Build history of the part. All positions in model axes, mm. A direction names the side the tool comes from. Coordinates: 2 decimals unless noted, no trailing zeros. Order: outer loops, then holes, each group sorted by start corner. A loop starts at its lowest first (then second) coordinate and runs counter-clockwise, first axis right, second up. Notation, with made-up numbers: (28.5, 6) - (77.5, 6) arc R14 ccw to (77.5, 25) - close; hole circle Ø11 at (17.25, -23.5). An arc over 180 degrees is marked (long way). One line per item, written item: value.
from build123d import *

# Parameters (mm, degrees)
F0_W     = 25.4
F0_H     = 50.8
F0_W_2   = 20.32
F0_H_2   = 45.72
F1_DEPTH = 304.8
F2_R     = 14.2875
F2_R_2   = 3.3782
F2_R_3   = 2.4892
F3_DEPTH = 25.4
F4_R     = 2.4892
F5_DEPTH = 50.801


with BuildPart() as f1:
    # F0 (on Top) → F1 (new body)
    with BuildSketch(Plane.XY):
        with Locations((12.7, -25.4)):
            Rectangle(F0_W, F0_H)
        with Locations((12.7, -25.4)):
            Rectangle(F0_W_2, F0_H_2, mode=Mode.SUBTRACT)
    extrude(amount=F1_DEPTH)

    # F2 (on face) → F3 (cut)
    with BuildSketch(Plane.YZ.offset(25.4)):
        with Locations((-25.4, 254)):
            Circle(F2_R)
        with Locations((-38.1, 38.1)):
            Circle(F2_R_2)
        with Locations((-38.1, 12.7)):
            Circle(F2_R_2)
        with Locations((-12.7, 38.1)):
            Circle(F2_R_2)
        with Locations((-12.7, 12.7)):
            Circle(F2_R_2)
        with BuildLine():
            ThreePointArc((-4.950288, 167.27389), (-8.392063, 169.573611), (-9.199618, 165.51376))
            ThreePointArc((-9.199618, 165.51376), (-6.486912, 164.974169), (-4.950288, 167.27389))
        make_face()
        with Locations((-43.360512, 131.352866)):
            Circle(F2_R_3)
        with BuildLine():
            Line((-25.4, 149.313378), (-11.1125, 149.313378))
            ThreePointArc((-11.1125, 149.313378), (-12.200071, 154.780968), (-15.297212, 159.416166))
            Line((-15.297212, 159.416166), (-25.4, 149.313378))
        make_face()
        with BuildLine():
            ThreePointArc((-15.297212, 159.416166), (-38.599929, 143.845789), (-11.1125, 149.313378))
            Line((-11.1125, 149.313378), (-25.4, 149.313378))
            Line((-25.4, 149.313378), (-15.297212, 159.416166))
        make_face()
    extrude(amount=-F3_DEPTH, mode=Mode.SUBTRACT)

    # F4 (on face) → F5 (cut, through all)
    with BuildSketch(Plane.XZ.offset(50.8)):
        with Locations((12.7, 292.1)):
            Circle(F4_R)
        with Locations((12.7, 266.7)):
            Circle(F4_R)
        with Locations((12.7, 241.3)):
            Circle(F4_R)
        with Locations((12.7, 215.9)):
            Circle(F4_R)
        with Locations((12.7, 190.5)):
            Circle(F4_R)
        with Locations((12.7, 165.1)):
            Circle(F4_R)
    extrude(amount=-F5_DEPTH, mode=Mode.SUBTRACT)


solid = f1.part
1. 3-axis set-ups, long thin cutter, end or side, ignore diameter. For faces 5 (the face through (13.849, -49.548, 213.692)), 6 (the face through (22.86, -41, 150)): which of +Z, -Z, +X, -X, +Y, -Y reach the whole face in a straight line?
Values found:
face 5: +Y, -Y
face 6: +Z, -Z
2. Probe line 1 along Z through (x, y) = (24.3, -25.4); line 2 along X through (y, z) = (-35, 240); line 3 along Z through (x, y) = (0.75, -12.7). List the from-to ranges inside material, lowest first.
Values found:
line 1: z = 0 to 135.03, 163.6 to 239.71, 268.29 to 304.8
line 2: x = 0 to 2.54, 22.86 to 25.4
line 3: z = 0 to 9.32, 16.08 to 34.72, 41.48 to 142.77, 155.86 to 247.45, 260.55 to 304.8
3. Band-saw the part on C-C, the plane z = 254. Give the cut face in (x, y).
Values found:
outline: (0, -50.8) - (25.4, -50.8) - (25.4, -39.69) - (22.86, -39.69) - (22.86, -48.26) - (2.54, -48.26) - (2.54, -39.69) - (0, -39.69) - close; (0, -11.11) - (2.54, -11.11) - (2.54, -2.54) - (22.86, -2.54) - (22.86, -11.11) - (25.4, -11.11) - (25.4, 0) - (0, 0) - close
4. Band-saw the part on B-B, the plane y = -25.4. Give the cut face in (x, z), and give its area (3 significant figures).
Values found:
outline: (0, 0) - (2.54, 0) - (2.54, 135.03) - (0, 135.03) - close; (0, 163.6) - (2.54, 163.6) - (2.54, 239.71) - (0, 239.71) - close; (0, 268.29) - (2.54, 268.29) - (2.54, 304.8) - (0, 304.8) - close; (22.86, 0) - (25.4, 0) - (25.4, 135.03) - (22.86, 135.03) - close; (22.86, 163.6) - (25.4, 163.6) - (25.4, 239.71) - (22.86, 239.71) - close; (22.86, 268.29) - (25.4, 268.29) - (25.4, 304.8) - (22.86, 304.8) - close
area: 1,260 mm2
5. Two-plate mould, pull along Y, no slides. Class faces 1 (the face through (12.16, -49.55, 238.87)), 2 (the face through (1.29, -13.43, 34.8)), 3 (the face through (13, 0, 150)), 4 (the face through (24.148, -15.381, 10.644)): pulls with the +Y half, pulls with the -Y half, needs draft (parallel to the pull), parting line crosses it, or undercut.
Values found:
face 1: needs draft
face 2: undercut
face 3: pulls with the +Y half
face 4: undercut
6. Band-saw the part on D-D, the plane z = 25. Give the cut face in (x, y), and give its area (3 significant figures).
Values found:
outline: (0, -50.8) - (25.4, -50.8) - (25.4, 0) - (0, 0) - close; hole (2.54, -48.26) - (22.86, -48.26) - (22.86, -2.54) - (2.54, -2.54) - close
area: 361 mm2
7. Band-saw the part on A-A, the plane x = 19.75. Give the cut face in (y, z), and give its area (3 significant figures).
Values found:
outline: (-50.8, 0) - (-48.26, 0) - (-48.26, 304.8) - (-50.8, 304.8) - close; (-2.54, 0) - (0, 0) - (0, 304.8) - (-2.54, 304.8) - close
area: 1,550 mm2
